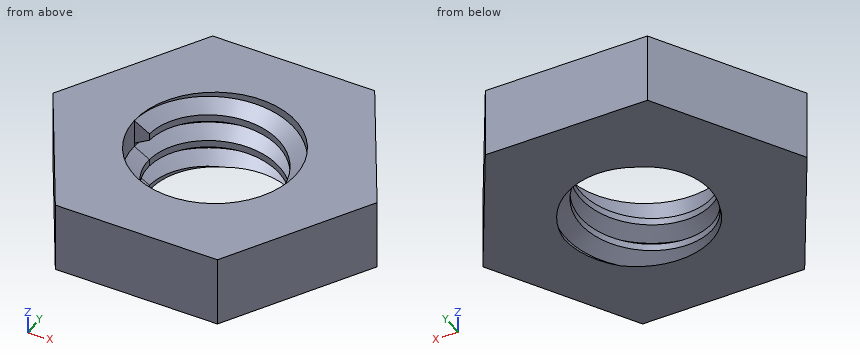
```python
from build123d import *

# Parameters (mm, degrees)
AUFSATZ_LINEAR_AUSTRAGEN1_DEPTH   = 5
GEWINDEBOHRUNG_F_R_PG7_F_HRUNG1_D = 11.5
GEWINDE1_PITCH                    = 2
SKIZZE12_W                        = 16.387995399
SKIZZE12_H                        = 16.357045455
SCHNITT_LINEAR_AUSTRAGEN1_DEPTH   = 10


with BuildPart() as part:
    # Skizze1 → Aufsatz-Linear austragen1 (new body)
    with BuildSketch(Plane.XY):
        Polygon((0, 0), (11.545, 0), (17.319505384, -10.001736713), (11.547005384, -20), (-0.002005384, -20), (-5.774505384, -10.001736713), align=None)
    extrude(amount=AUFSATZ_LINEAR_AUSTRAGEN1_DEPTH)

    # Gewindebohrung für Pg7 Führung1 (through all)
    with Locations(Plane(origin=(5.771497308, -10, 5), x_dir=(1, 0, 0), z_dir=(0, 0, 1))):
        with Locations((0, 0)):
            Hole(GEWINDEBOHRUNG_F_R_PG7_F_HRUNG1_D / 2)

    # Gewinde1: the profile of Gewindeprofil2 profile screwed along a right-hand helix of 5 turns, 10 arcs to a turn; built about Z, then put on its axis
    gewinde1_z = Axis((0, 0, 0), (0, 0, 1))
    gewinde1_corners = [(5.7503, 0, -0.000173205), (5.7503, 0, 1.7501732), (4.66746825, 0, 1.124999997), (4.66746825, 0, 0.624999997)]
    with BuildLine(mode=Mode.PRIVATE) as gewinde1_profile:
        Line(gewinde1_corners[0], gewinde1_corners[1])
        Line(gewinde1_corners[1], gewinde1_corners[2])
        Line(gewinde1_corners[2], gewinde1_corners[3])
        Line(gewinde1_corners[3], gewinde1_corners[0])
    gewinde1_cap = Face(gewinde1_profile.wire())
    gewinde1_turn_angles = [0, 18, 36, 54, 72, 90, 108, 126, 144, 162, 180, 198, 216, 234, 252, 270, 288, 306, 324, 342, 360]
    gewinde1_turn_weights = [1, 0.9510565162951535, 1, 0.9510565162951535, 1, 0.9510565162951535, 1, 0.9510565162951535, 1, 0.9510565162951535, 1, 0.9510565162951535, 1, 0.9510565162951535, 1, 0.9510565162951535, 1, 0.9510565162951535, 1, 0.9510565162951535, 1]
    gewinde1_turn_rails = [Edge.make_bspline([Vector(p[0], p[1], 0).rotate(gewinde1_z, gewinde1_turn_angles[k]) / gewinde1_turn_weights[k] + Vector(0, 0, p[2] + GEWINDE1_PITCH * gewinde1_turn_angles[k] / 360) for k in range(21)], [0, 0, 0, 1, 1, 2, 2, 3, 3, 4, 4, 5, 5, 6, 6, 7, 7, 8, 8, 9, 9, 10, 10, 10], 2, gewinde1_turn_weights) for p in gewinde1_corners]
    gewinde1_turn_sides = [Face.make_surface_from_curves(gewinde1_turn_rails[p[0]], gewinde1_turn_rails[p[1]]) for p in [(0, 1), (1, 2), (2, 3), (3, 0)]]
    gewinde1 = Plane(origin=(5.771497308, -10, 5), x_dir=(-1, 0, 0), z_dir=(0, 0, -1)) * Solid(Shell([*[p.moved(Location((0, 0, GEWINDE1_PITCH * i))) for i in range(5) for p in gewinde1_turn_sides], gewinde1_cap, gewinde1_cap.rotate(gewinde1_z, 1800).moved(Location((0, 0, GEWINDE1_PITCH * 1800 / 360)))]))
    add(gewinde1)

    # Skizze12 → Schnitt-Linear austragen1 (cut)
    with BuildSketch(Plane(origin=(0, 0, 0), x_dir=(-1, 0, 0), z_dir=(0, 0, -1))):
        with Locations((-5.65643771, -10.147012235)):
            Rectangle(SKIZZE12_W, SKIZZE12_H)
    extrude(amount=SCHNITT_LINEAR_AUSTRAGEN1_DEPTH, mode=Mode.SUBTRACT)


solid = part.part
```
Here's how the part is built. I have some questions about the finished solid (model axes, mm). Coordinates: 2 decimals unless noted, no trailing zeros. Write each loop counter-clockwise with the first axis right and the second up, starting at its lowest first coordinate (ties: lowest second). Pieces come first, ordered by that corner, then holes. Notation, with made-up numbers: (-26.5, 87.25) - (28.5, 87.25) arc R7 cw to (28.5, 91.25) - close; hole circle Ø6 at (59.5, 9.5). An arc over 180 degrees is marked (long way). One line per item, written item: value.
1) Suppose I cut it at A-A on x = 15.75. Write out the boundary of the cut face in (y, z), and give its area (3 significant figures).
Model answer:
outline: (-12.72, 0) - (-7.28, 0) - (-7.28, 5) - (-12.72, 5) - close
area: 27.2 mm²
2) I'm going to push flat-ended pins straight in: P1, Ø1.5, axis at x = 5.5, z = 1.5, coming from the +Y side; P2, Ø1, axis at y = -13, z = 3.5, coming from the -X side; P3, Ø1.5, axis at y = -4.5, z = 3.5, coming from the +X side; P4, Ø1.5, axis at y = -5, z = 2, coming from the -X side. Where does each tip first touch, or does it pass through?
Model answer:
P1: stops at y = 0
P2: stops at x = -4.33
P3: stops at x = 14.58
P4: stops at x = -3.32
3) Suppose I cut it at B-B on y = -16.5. Write out the boundary of the cut face in (x, z).
Model answer:
outline: (-2.02, 0) - (13.57, 0) - (13.57, 5) - (-2.02, 5) - close
4) I need wall thicknesses on line 1 along Y through (x, z) = (6.5, 0.85); line 2 along Z through (x, y) = (3, -5); line 3 along X through (y, z) = (-13.75, 3.85). Which ranges of each line are inside material? Lowest first, please.
Model answer:
line 1: y = -20 to -14.61, -4.55 to 0
line 2: z = 0 to 0.64, 0.93 to 2.64, 2.93 to 4.64
line 3: x = -3.61 to 1.41, 10.13 to 15.16
